```python
from build123d import *

# Parameters (mm, degrees)
F0_W     = 60
F0_H     = 20
F1_DEPTH = 5
F3_DEPTH = 20
F5_D     = 5
F7_D     = 5


# Not quite as in the source:
# - a pattern or mirror of a feature is missing from the dataset's text; its kind, count and spacing are read off the source's solid


with BuildPart() as f1:
    # F0 (on Top) → F1 (new body)
    with BuildSketch(Plane.XY):
        Rectangle(F0_W, F0_H)
    extrude(amount=F1_DEPTH)

    # F2 (on face) → F3 (join)
    with BuildSketch(Plane.XY.offset(5)):
        Polygon((-15, 10), (-15, -10), (-10, -10), (-10, 5), (0, 5), (0, 10), align=None)
    f3 = extrude(amount=F3_DEPTH)

    # F3_copies: F3 across plane
    add(f3.mirror(Plane(origin=(0, 0, 0), x_dir=(0, 0, 1), z_dir=(1, 0, 0))))

    # F5 (through all)
    with Locations(Plane.XY.offset(5)):
        with Locations((-25, 0)):
            f5 = Hole(F5_D / 2)

    # F5_copies: F5 across plane
    add(f5.mirror(Plane(origin=(0, 0, 0), x_dir=(0, 0, 1), z_dir=(1, 0, 0))), mode=Mode.SUBTRACT)

    # F7 (through all)
    with Locations(Plane.XZ.offset(-5)):
        with Locations((0, 15)):
            Hole(F7_D / 2)


solid = f1.part
```
Part model, mm, in its own coordinate system. A direction names the side the tool comes from. Coordinates: 2 decimals unless noted, no trailing zeros. Loops run counter-clockwise (first coordinate to the right, second up) from the corner with the lowest first, then second, coordinate; pieces in that order, holes last. Notation, with made-up numbers: (-40, 80) - (-3, 80) arc R19 cw to (-3, 114) - close; hole circle Ø2 at (63.25, -22). An arc over 180 degrees is marked (long way). Write item = value, one per line. Start each with the question number.
Item 1: Mould opens along X. For faces 6 (the flat face through (4, 7, 25)), 7 (the flat face through (0, -2, 5)), 8 (the flat face through (15, 0, 15)) say: released by +X, released by -X, zero draft, split by the parting line, or undercut.
Item 2: Flat gauge pins, fed straight in: pin 1 Ø7.5 at (y, z) = (0.5, 13.5) entering from -X; pin 2 Ø3 at (x, z) = (0, 15) entering from -Y; pin 3 Ø10 at (y, z) = (-3, 12.5) entering from +X; pin 4 Ø1 at (x, z) = (7.5, 19) entering from -Y. Where does each tip first touch, or does it go through?
Item 3: Cut at B-B, the plane z = 15. Give the cut face in (x, y).
Item 4: Wall check: L1, parallel to X at y = 4.5, z = 21.5; L2, parallel to Y at x = -25, z = 2.5; L3, parallel to Z at x = 0, y = 6. Give the ranges that are in metal, low to high. Write a range as from..to.
Item 5: Cut at C-C, the plane x = 25. Give the cut face in (y, z).
Item 6: 3-axis set-ups, long thin cutter, end or side, ignore diameter. For faces 1 (the flat face through (0, -10, 4)), 2 (the flat face through (-21, 0, 5)), 3 (the cylindrical face through (22.5, 0.1, 2.5)), 4 (the flat face through (22, 0, 5)), 5 (the flat face through (10, -3, 15)): which of +Z, -Z, +X, -X, +Y, -Y reach the whole face in a straight line?
Item 7: Cut at D-D, the plane y = 6.5. Give the cut face in (x, z).
Item 8: Cut at A-A, the plane y = -1.5. Give the cut face in (x, z), and give its area (3 significant figures).
The answers:
q1.face_6 = zero draft
q1.face_7 = undercut
q1.face_8 = released by +X
q2.pin_1 = -15
q2.pin_2 = through
q2.pin_3 = 15
q2.pin_4 = 5
q3.outline = (-15, -10) - (-10, -10) - (-10, 5) - (-2.5, 5) - (-2.5, 10) - (-15, 10) - close; (2.5, 5) - (10, 5) - (10, -10) - (15, -10) - (15, 10) - (2.5, 10) - close
q4.L1 = -15..-10, 10..15
q4.L2 = -10..-2.5, 2.5..10
q4.L3 = 0..12.5, 17.5..25
q5.outline = (-10, 0) - (-2.5, 0) - (-2.5, 5) - (-10, 5) - close; (2.5, 0) - (10, 0) - (10, 5) - (2.5, 5) - close
q6.face_1 = +Z, -Z, +X, -X, -Y
q6.face_2 = +Z, -X, +Y, -Y
q6.face_3 = +Z, -Z
q6.face_4 = +Z, +X, +Y, -Y
q6.face_5 = +Z, -Y
q7.outline = (-30, 0) - (30, 0) - (30, 5) - (15, 5) - (15, 25) - (-15, 25) - (-15, 5) - (-30, 5) - close; hole circle Ø5 at (0, 15)
q8.outline = (-30, 0) - (-27, 0) - (-27, 5) - (-30, 5) - close; (-23, 0) - (23, 0) - (23, 5) - (15, 5) - (15, 25) - (10, 25) - (10, 5) - (-10, 5) - (-10, 25) - (-15, 25) - (-15, 5) - (-23, 5) - close; (27, 0) - (30, 0) - (30, 5) - (27, 5) - close
q8.area = 460 mm2
